```python
from build123d import *

# Parameters (mm, degrees)
BOSS_EXTRUDE1_DEPTH      = 3
BOSS_EXTRUDE2_DEPTH      = 24.22
BOSS_EXTRUDE2_DEPTH_BACK = 24.22
SKETCH4_W                = 39.44
SKETCH4_H                = 18
CUT_EXTRUDE2_DEPTH       = 49.314655701
FILLET1_R                = 3
FILLET2_R                = 3
FILLET3_R                = 4


with BuildPart() as part:
    # Sketch1 → Boss-Extrude1 (new body)
    with BuildSketch(Plane(origin=(0, 0, 0), x_dir=(1, 0, 0), z_dir=(0, 1, 0))):
        with BuildLine():
            ThreePointArc((-2, 18.983932023), (-1.070466269, 18.417482923), (0, 18.22))
            Line((0, 18.22), (0, -18.22))
            ThreePointArc((0, -18.22), (-1.070466269, -18.417482923), (-2, -18.983932023))
            ThreePointArc((-2, -18.983932023), (-2.802517077, -22.290466269), (0, -24.22))
            Line((0, -24.22), (3, -24.22))
            Line((3, -24.22), (3, 24.22))
            Line((3, 24.22), (0, 24.22))
            ThreePointArc((0, 24.22), (-2.802517077, 22.290466269), (-2, 18.983932023))
        make_face()
        with BuildLine():
            ThreePointArc((0.787400787, -19.77), (1.41804642, -20.376409845), (1.65, -21.22))
            ThreePointArc((1.65, -21.22), (-0.843590155, -22.63804642), (-0.787400787, -19.77))
            ThreePointArc((-0.787400787, -19.77), (-0.370606333, -19.500307136), (0, -19.17))
            ThreePointArc((0, -19.17), (0.370606333, -19.500307136), (0.787400787, -19.77))
        make_face(mode=Mode.SUBTRACT)
        with BuildLine():
            ThreePointArc((0.787400787, 22.67), (1.41804642, 22.063590155), (1.65, 21.22))
            ThreePointArc((1.65, 21.22), (-0.843590155, 19.80195358), (-0.787400787, 22.67))
            ThreePointArc((-0.787400787, 22.67), (-0.370606333, 22.939692864), (0, 23.27))
            ThreePointArc((0, 23.27), (0.370606333, 22.939692864), (0.787400787, 22.67))
        make_face(mode=Mode.SUBTRACT)
    extrude(amount=BOSS_EXTRUDE1_DEPTH)

    # Sketch2 → Boss-Extrude2 (add, two sides: drawn at the far end of the back side and taken through both)
    with BuildSketch(Plane.XY.offset(-BOSS_EXTRUDE2_DEPTH_BACK)):
        Polygon((3, 3), (3, 0), (10.137467504, 0), (27.546655814, 17.409188309), (25.595041097, 19.360803025), (12.867119036, 6.632880964), (4, 15.5), (16.727922061, 28.227922061), (14.776307345, 30.179536777), (2.048385284, 17.451614716), (0.634171722, 18.865828278), (-1.487148622, 16.744507935), (6, 9.257359313), (6, 3), align=None)
    extrude(amount=BOSS_EXTRUDE2_DEPTH + BOSS_EXTRUDE2_DEPTH_BACK)

    # Sketch4 → Cut-Extrude2 (cut, through all)
    with BuildSketch(Plane(origin=(-7.701614716, 7.701614716, 0), x_dir=(0, 0, 1), z_dir=(-0.7071067811865439, 0.7071067811865511, 0))):
        with Locations((0, 22.788582233)):
            Rectangle(SKETCH4_W, SKETCH4_H)
    extrude(amount=-CUT_EXTRUDE2_DEPTH, mode=Mode.SUBTRACT)

    # Fillet1
    fillet1_edges = [part.edges().sort_by_distance(p)[0] for p in [
        (6, 3, 0),
        (6, 9.257359313, 0),
    ]]
    fillet(fillet1_edges, radius=FILLET1_R)

    # Fillet2
    fillet2_edges = [part.edges().sort_by_distance(p)[0] for p in [
        (-1.487148622, 16.744507935, 0),
        (10.137467504, 0, 0),
    ]]
    fillet(fillet2_edges, radius=FILLET2_R - 0.0001)  # a hair under: the kernel refuses the full size

    # Fillet3
    fillet3_edges = [part.edges().sort_by_distance(p)[0] for p in [
        (4, 15.5, -21.97),
        (4, 15.5, 21.97),
    ]]
    fillet(fillet3_edges, radius=FILLET3_R)


solid = part.part
```
Geometry check sheet. Reference: the model listing, model coordinates, mm. A direction names the side the tool comes from. Round coordinates to 2 decimals unless told otherwise and drop trailing zeros. Order: outer loops, then holes, each group sorted by start corner. A loop starts at its lowest first (then second) coordinate and runs counter-clockwise, first axis right, second up. Notation, with made-up numbers: M 63,-19 L 122,-19 A28 ccw 122,17 Z; hole C -23.75,55 d5. An arc over 180 degrees is marked long. Write item = value, one per line.
Q1. Set-up check for faces 5 (the flat face through (26.585, 18.371, -22.002)), 6 (the flat face through (6, 7, 0)), 7 (the flat face through (19.32, 13.086, -22.002)): record each of +Z, -Z, +X, -X, +Y, -Y from which the full face is reachable in a straight line by a thin tool's end or side.
Answer block:
face_5 = +Z, -Z, +X, +Y
face_6 = +Z, -Z, -X
face_7 = +Z, -Z
Q2. Depth check by flat-ended pin: pin 1 Ø0.6 at (y, z) = (6.5, 4) entering from -X; pin 2 Ø10 at (y, z) = (21, 12.5) entering from -X; pin 3 Ø3 at (x, z) = (0.5, -0.5) entering from +Y; pin 4 Ø2 at (x, y) = (15.5, 25) entering from -Z. Enter the tip coordinate at first touch or a pass-through.
Answer block:
pin_1 = 6
pin_2 = -0.24
pin_3 = 18.87
pin_4 = through
Q3. Section check D-D (y = 11). Enter the section's corners in (x, z).
Answer block:
outline = M 4.26,-24.22 L 8.5,-24.22 L 8.5,24.22 L 4.26,24.22 Z; M 17.23,-24.22 L 21.14,-24.22 L 21.14,-19.72 L 17.23,-19.72 Z; M 17.23,19.72 L 21.14,19.72 L 21.14,24.22 L 17.23,24.22 Z
Q4. Section check A-A (y = 24.5). Enter the section's corners in (x, z).
Answer block:
outline = M 9.1,-24.22 L 13,-24.22 L 13,-19.72 L 9.1,-19.72 Z; M 9.1,19.72 L 13,19.72 L 13,24.22 L 9.1,24.22 Z
Q5. Release check for a two-part mould opening along Z. For faces 1 (the flat face through (8, 11, 24.22)), 2 (the flat face through (13.66, 3.52, -0.34)), 3 (the flat face through (20, 12, -19.72)), 4 (the flat face through (0, 1, 0)) record: released by +Z, released by -Z, zero draft, split by the parting line, or undercut.
Answer block:
face_1 = released by +Z
face_2 = zero draft
face_3 = undercut
face_4 = undercut
Q6. Scan lines: line 1 (Z direction, x = 4.5, y = 19); line 2 (Y direction, x = 2, z = 16.5); line 3 (X direction, y = 1, z = -21). Record each from-to range of solid material in increasing order.
Answer block:
line_1 = -24.22 to -19.72, 19.72 to 24.22
line_2 = 0 to 3, 13.26 to 17.5
line_3 = -2.99 to -1.64, 1.64 to 11.14
Q7. Section check B-B (x = 18.5). Enter the section's corners in (y, z), plus the area to 3 significant figures.
Answer block:
outline = M 8.36,-24.22 L 12.27,-24.22 L 12.27,-19.72 L 8.36,-19.72 Z; M 8.36,19.72 L 12.27,19.72 L 12.27,24.22 L 8.36,24.22 Z
area = 35.1 mm^2
